Part model, mm, in its own coordinate system. A direction names the side the tool comes from. Round coordinates to 2 decimals unless told otherwise and drop trailing zeros. Write each loop counter-clockwise with the first axis right and the second up, starting at its lowest first coordinate (ties: lowest second). Pieces come first, ordered by that corner, then holes.
from build123d import *

# Parameters (mm, degrees)
CROQUIS1_W              = 68
CROQUIS1_H              = 88
CROQUIS1_W_2            = 60
CROQUIS1_H_2            = 80
SALIENTE_EXTRUIR1_DEPTH = 27
CROQUIS3_W              = 68
CROQUIS3_H              = 88
SALIENTE_EXTRUIR2_DEPTH = 3
CROQUIS4_W              = 67
CROQUIS4_H              = 5
CORTAR_EXTRUIR1_DEPTH   = 69
CROQUIS5_W              = 55
CROQUIS5_H              = 5
CORTAR_EXTRUIR2_DEPTH   = 89


with BuildPart() as part:
    # Croquis1 → Saliente-Extruir1 (new body)
    with BuildSketch(Plane(origin=(0, 0, 0), x_dir=(1, 0, 0), z_dir=(0, 1, 0))):
        with Locations((30, 40)):
            Rectangle(CROQUIS1_W, CROQUIS1_H)
        with Locations((30, 40)):
            Rectangle(CROQUIS1_W_2, CROQUIS1_H_2, mode=Mode.SUBTRACT)
    extrude(amount=SALIENTE_EXTRUIR1_DEPTH)

    # Croquis3 → Saliente-Extruir2 (add)
    with BuildSketch(Plane(origin=(0, 27, 0), x_dir=(1, 0, 0), z_dir=(0, 1, 0))):
        with Locations((30, 40)):
            Rectangle(CROQUIS3_W, CROQUIS3_H)
    extrude(amount=SALIENTE_EXTRUIR2_DEPTH)

    # Croquis4 → Cortar-Extruir1 (cut, through all)
    with BuildSketch(Plane.ZY.offset(4)):
        with Locations((-40, 17.5)):
            Rectangle(CROQUIS4_W, CROQUIS4_H)
    extrude(amount=-CORTAR_EXTRUIR1_DEPTH, mode=Mode.SUBTRACT)

    # Croquis5 → Cortar-Extruir2 (cut, through all)
    with BuildSketch(Plane.XY.offset(4)):
        with Locations((30, 17.5)):
            Rectangle(CROQUIS5_W, CROQUIS5_H)
    extrude(amount=-CORTAR_EXTRUIR2_DEPTH, mode=Mode.SUBTRACT)


solid = part.part
Q1. Two-plate mould, pull along Z, no slides. Class faces 1 (the flat face through (30, 20, -82)), 2 (the flat face through (29.5, 14.8, 4)), 3 (the flat face through (-2, 17, -73.5)): released by +Z, released by -Z, zero draft, split by the parting line, or undercut.
Q2. Saw through at D-D, the plane y = 26. Write the cut outline in (x, z), and give its area (3 significant figures).
Q3. Wall check: line 1 (X direction, y = 4.5, z = -7); line 2 (Z direction, x = 7, y = 4.5); line 3 (Y direction, x = 7, z = -2). Give the ranges that are in metal, low to high.
Q4. Tool access for faces 4 (the flat face through (2.5, 17, 2)), 5 (the flat face through (30, 13, -80)), 6 (the flat face through (-2, 15, -40)), 7 (the flat face through (-4, 14.8, -39.4)): list every direction of +Z, -Z, +X, -X, +Y, -Y with a clear straight run to the whole face (end or side of a thin tool).
Q5. Saw through at B-B, the plane z = -62. Write the cut outline in (x, y).
Q6. Saw through at C-C, the plane x = 37. Write the cut outline in (y, z), and give its area (3 significant figures).
Q7. Saw through at A-A, the plane y = 17.25. Write the cut outline in (x, z), and give its area (3 significant figures).
Computed:
1. face 1: zero draft
1. face 2: released by +Z
1. face 3: undercut
2. outline: (-4, -84) - (64, -84) - (64, 4) - (-4, 4) - close; hole (0, -80) - (60, -80) - (60, 0) - (0, 0) - close
2. area: 1,180 mm2
3. line 1: x = -4 to 0, 60 to 64
3. line 2: z = -84 to -80, 0 to 4
3. line 3: y = 27 to 30
4. face 4: +Z, -Z
4. face 5: -Y
4. face 6: +X, -X
4. face 7: +Z, -Z, -X, +Y, -Y
5. outline: (-4, 0) - (0, 0) - (0, 15) - (-4, 15) - close; (-4, 20) - (0, 20) - (0, 27) - (60, 27) - (60, 20) - (64, 20) - (64, 30) - (-4, 30) - close; (60, 0) - (64, 0) - (64, 15) - (60, 15) - close
6. outline: (0, -84) - (15, -84) - (15, -80) - (0, -80) - close; (0, 0) - (15, 0) - (15, 4) - (0, 4) - close; (20, -84) - (30, -84) - (30, 4) - (20, 4) - (20, 0) - (27, 0) - (27, -80) - (20, -80) - close
6. area: 440 mm2
7. outline: (-4, -84) - (2.5, -84) - (2.5, -80) - (0, -80) - (0, -73.5) - (-4, -73.5) - close; (-4, -6.5) - (0, -6.5) - (0, 0) - (2.5, 0) - (2.5, 4) - (-4, 4) - close; (57.5, -84) - (64, -84) - (64, -73.5) - (60, -73.5) - (60, -80) - (57.5, -80) - close; (57.5, 0) - (60, 0) - (60, -6.5) - (64, -6.5) - (64, 4) - (57.5, 4) - close
7. area: 208 mm2
